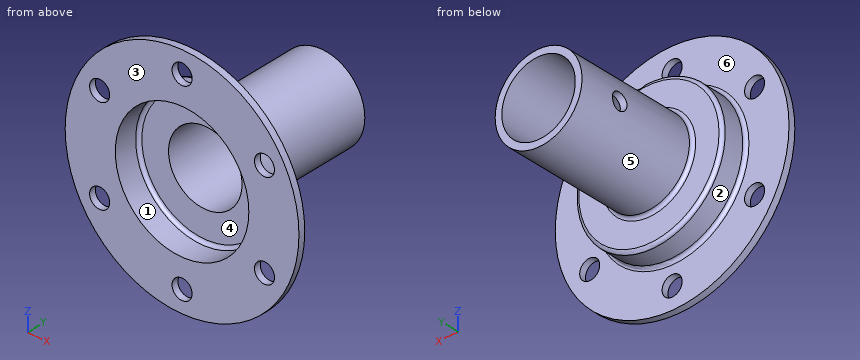
```python
from build123d import *

# Parameters (mm, degrees)
SKETCH_2_R          = 3
CUT_EXTRUDE_1_DEPTH = 3
SKETCH_3_R          = 2.5
CUT_EXTRUDE_2_DEPTH = 36


with BuildPart() as part:
    # 草图1 → 旋转1 (revolve)
    with BuildSketch(Plane.XY):
        with BuildLine():
            Line((20, 0), (35, 0))
            Line((35, 0), (35, 2))
            Line((35, 2), (23, 2))
            ThreePointArc((23, 2), (22.292893219, 2.292893219), (22, 3))
            Line((22, 3), (22, 9))
            ThreePointArc((22, 9), (21.707106781, 9.707106781), (21, 10))
            Line((21, 10), (14, 10))
            ThreePointArc((14, 10), (13.292893219, 10.292893219), (13, 11))
            Line((13, 11), (13, 48))
            Line((13, 48), (11, 48))
            Line((11, 48), (11, 8))
            Line((11, 8), (19, 8))
            ThreePointArc((19, 8), (19.707106781, 7.707106781), (20, 7))
            Line((20, 7), (20, 0))
        make_face()
    revolve(axis=Axis((0, 0, 0), (0, 1, 0)))

    # 草图2 → 切除-拉伸1 (cut, through all)
    with BuildSketch(Plane(origin=(0, 2, 0), x_dir=(1, 0, 0), z_dir=(0, 1, 0))):
        with Locations((0, 28.5)):
            Circle(SKETCH_2_R)
        with Locations((24.681724008, 14.25)):
            Circle(SKETCH_2_R)
        with Locations((24.681724008, -14.25)):
            Circle(SKETCH_2_R)
        with Locations((0, -28.5)):
            Circle(SKETCH_2_R)
        with Locations((-24.681724008, -14.25)):
            Circle(SKETCH_2_R)
        with Locations((-24.681724008, 14.25)):
            Circle(SKETCH_2_R)
    extrude(amount=-CUT_EXTRUDE_1_DEPTH, mode=Mode.SUBTRACT)

    # 草图3 → 切除-拉伸2 (cut, through all)
    with BuildSketch(Plane(origin=(0, 0, 0), x_dir=(0, 0, -1), z_dir=(1, 0, 0))):
        with Locations((0, 35)):
            Circle(SKETCH_3_R)
    extrude(amount=-CUT_EXTRUDE_2_DEPTH, mode=Mode.SUBTRACT)


solid = part.part
```
For this review, take the finished solid that the model builds, in its own axes (mm). Face numbers are marked on the shaded views. A direction names the side the tool comes from. Coordinates: 2 decimals unless noted, no trailing zeros. Write each loop counter-clockwise with the first axis right and the second up, starting at its lowest first coordinate (ties: lowest second). Pieces come first, ordered by that corner, then holes. Notation, with made-up numbers: (70.5, 29.25) -> (90.5, 29.25) arc R7 cw to (90.5, 38.25) -> close; hole circle Ø1 at (59, 83.25). An arc over 180 degrees is marked (long way). Put each result on its own line as item: value.
Q1. The part is to be moulded in two halves that separate along Z. For the marked faces 4, 5 and 6, say which applies: +Z half, -Z half, draft (parallel to the pull), parting line (faces both ways), or undercut.
From the geometry:
face 4: undercut
face 5: parting line
face 6: draft
Q2. Take a section at B-B, the plane z = 28.5. State the section outline as (x, y) points, then the cut area to 3 significant figures.
From the geometry:
outline: (-20.32, 0) -> (-3, 0) -> (-3, 2) -> (-20.32, 2) -> close; (3, 0) -> (20.32, 0) -> (20.32, 2) -> (3, 2) -> close
area: 69.3 mm2
Q3. Take a section at A-A, the plane z = 0. Count the separate pieces of the cut face and the enclosed holes in it, then the cut area to 3 significant figures.
From the geometry:
separate pieces: 3
enclosed holes: 0
area: 271 mm2
Q4. Clearance check with flat-ended pins moving along their axes: pin 1 Ø9.5 at (x, z) = (-24.68, 14.25) entering from -Y; pin 2 Ø11.5 at (x, z) = (-8.5, 8) entering from -Y; pin 3 Ø4 at (y, z) = (35, 0) entering from -X. State where each tip first meets the part, or that it passes through.
From the geometry:
pin 1: stops at y = 0
pin 2: stops at y = 8
pin 3: stops at x = 10.82
Q5. Wall thickness on L1, parallel to Z at x = 0, y = 1.1; L2, parallel to Z at x = 0, y = 3; L3, parallel to X at y = 0.55, z = -14.25: over which ranges is each line inside the solid? List them lowest first.
From the geometry:
L1: z = -35 to -31.5, -25.5 to -20, 20 to 25.5, 31.5 to 35
L2: z = -22 to -20, 20 to 22
L3: x = -31.97 to -27.68, -21.68 to -14.03, 14.03 to 21.68, 27.68 to 31.97
Q6. Take a section at C-C, the plane x = 25.5. State the section outline as (y, z) points.
From the geometry:
outline: (0, -23.97) -> (2, -23.97) -> (2, -17.14) -> (0, -17.14) -> close; (0, -11.36) -> (2, -11.36) -> (2, 11.36) -> (0, 11.36) -> close; (0, 17.14) -> (2, 17.14) -> (2, 23.97) -> (0, 23.97) -> close
Q7. Take a section at D-D, the plane y = 24. State the section outline as (x, z) points, then the cut area to 3 significant figures.
From the geometry:
outline: circle Ø26 at (0, 0); hole circle Ø22 at (0, 0)
area: 151 mm2
Q8. Tool access review of the marked faces 1, 2 and 3: name each direction out of +Z, -Z, +X, -X, +Y, -Y from which nothing blocks a thin tool from reaching the whole face with its end or side.
From the geometry:
face 1: -Y
face 2: +Y
face 3: +Z, -Z, +X, -X, -Y
